Solid Edge part; units mm, degrees
sketch "Sketch1" plane through (0, 0, 0) normal (0, -1, 0) x (1, 0, 0)
  line L0 (4.2, 4.5) -> (0, 4.5)
  line L1 (0, 4.5) -> (0, 8.5)
  line L2 (0, 8.5) -> (1.2, 8.5)
  line L3 (1.2, 8.5) -> (1.2, 6.5)
  line L4 (1.2, 6.5) -> (4.2, 6.5)
  line L5 (4.2, 6.5) -> (4.2, 4.5)
revolve "RevolvedProtrusion1" add sketch "Sketch1" angle 360 about axis through (0, 0, 0) along (1, 0, 0)
chamfer "Chamfer1" distance 0.2 angle 45 1 edges at (4.2, 0, -6.5)
Build history of the part. All positions in model axes, mm. A direction names the side the tool comes from. Round coordinates to 2 decimals unless told otherwise and drop trailing zeros. Write each loop counter-clockwise with the first axis right and the second up, starting at its lowest first coordinate (ties: lowest second). Pieces come first, ordered by that corner, then holes. Notation, with made-up numbers: M 27,25 L 52,25 A37 cw 52,63 Z; hole C 86.25,89.25 d1. An arc over 180 degrees is marked long. Answer in a Markdown table with one row per item.
1. Saw through at A-A (z = 0). List the corners of the cut face in (x, y).
Geometry check:
| item | result |
|---|---|
| outline | M 0,-8.5 L 1.2,-8.5 L 1.2,-6.5 L 4,-6.5 L 4.2,-6.3 L 4.2,-4.5 L 0,-4.5 Z; M 0,4.5 L 4.2,4.5 L 4.2,6.3 L 4,6.5 L 1.2,6.5 L 1.2,8.5 L 0,8.5 Z |
2. Saw through at D-D (z = 7.5). List the corners of the cut face in (x, y).
Geometry check:
| item | result |
|---|---|
| outline | M 0,-4 L 1.2,-4 L 1.2,4 L 0,4 Z |
3. Flat gauge pins, fed straight in: P1, Ø2, axis at x = 3.5, z = -6.5, coming from the -Y side; P2, Ø1.5, axis at x = 0.5, y = -5, coming from the -Z side. Where does each tip first touch, or does it go through?
Geometry check:
| item | result |
|---|---|
| P1 | y = -3.46 |
| P2 | z = -7.36 |
4. Probe L1, parallel to Y at x = 1, z = 0; L2, parallel to Y at x = 1.7, z = 0. List the from-to ranges inside material, lowest first. Write a range as [from, to].
Geometry check:
| item | result |
|---|---|
| L1 | [-8.5, -4.5], [4.5, 8.5] |
| L2 | [-6.5, -4.5], [4.5, 6.5] |
5. Mould opens along Y. For faces 3 (the face through (4.2, 3, 4)), 4 (the face through (2.07, 4.46, -0.59)), 5 (the face through (0.608, -7.167, 4.57)) say: +Y half, -Y half, draft (parallel to the pull), parting line (faces both ways), or undercut.
Geometry check:
| item | result |
|---|---|
| face 3 | draft |
| face 4 | undercut |
| face 5 | parting line |
6. Which spindle directions (+Z, -Z, +X, -X, +Y, -Y) get a long thin tool onto all of the face, cutting with end or side? Do faces 1 (the face through (1.2, 5, 4.4)), 2 (the face through (0, 4, 4)). Say none if no direction does.
Geometry check:
| item | result |
|---|---|
| face 1 | +X |
| face 2 | +Z, -Z, -X, +Y, -Y |
7. Saw through at C-C (x = 0.7). List the corners of the cut face in (y, z).
Geometry check:
| item | result |
|---|---|
| outline | C 0,0 d17; hole C 0,0 d9 |
